Here's the drawing with two shaded views (mm, measured from the low corner). I have some questions. A direction names the side the tool comes from. Round coordinates to 2 decimals unless told otherwise and drop trailing zeros. Order: outer loops, then holes, each group sorted by start corner. A loop starts at its lowest first (then second) coordinate and runs counter-clockwise, first axis right, second up.
Q1. Will these pins go through, and if not, where does the flat tip stop? P1, Ø6.5, axis at x = 14.5, z = 74, coming from the +Y side; P2, Ø20.5, axis at y = 65.5, z = 60.5, coming from the +X side; P3, Ø11, axis at x = 93, y = 63.5, coming from the +Z side.
Q2. If we section it at A-A (z = 94): Please give me the cut outline in (x, y).
Q3. If we section it at D-D (x = 32.5): Please give me the cut outline in (y, z).
Q4. We'd pull the mould along X, two halves only. Please class the marked faces 1, 2 and 3: pulls with the +X half, pulls with the -X half, needs draft (parallel to the pull), parting line crosses it, or undercut.
Q5. For the marked faces 4 and 5, which set-ups out of +Z, -Z, +X, -X, +Y, -Y let a thin tool reach every point of the face, with its end or its side?
Q6. If we section it at C-C (x = 50.8): Please give me the cut outline in (y, z), plus the area to 3 significant figures.
Q7. If we section it at B-B (x = 89): Please give me the cut outline in (y, z).
Q8. If I drill on line 1 (X direction, y = 53, z = 64); line 2 (Y direction, x = 15, z = 39); line 3 (X direction, y = 70, z = 19.5), over which ranges is the centre line in solid material (lowest first)?
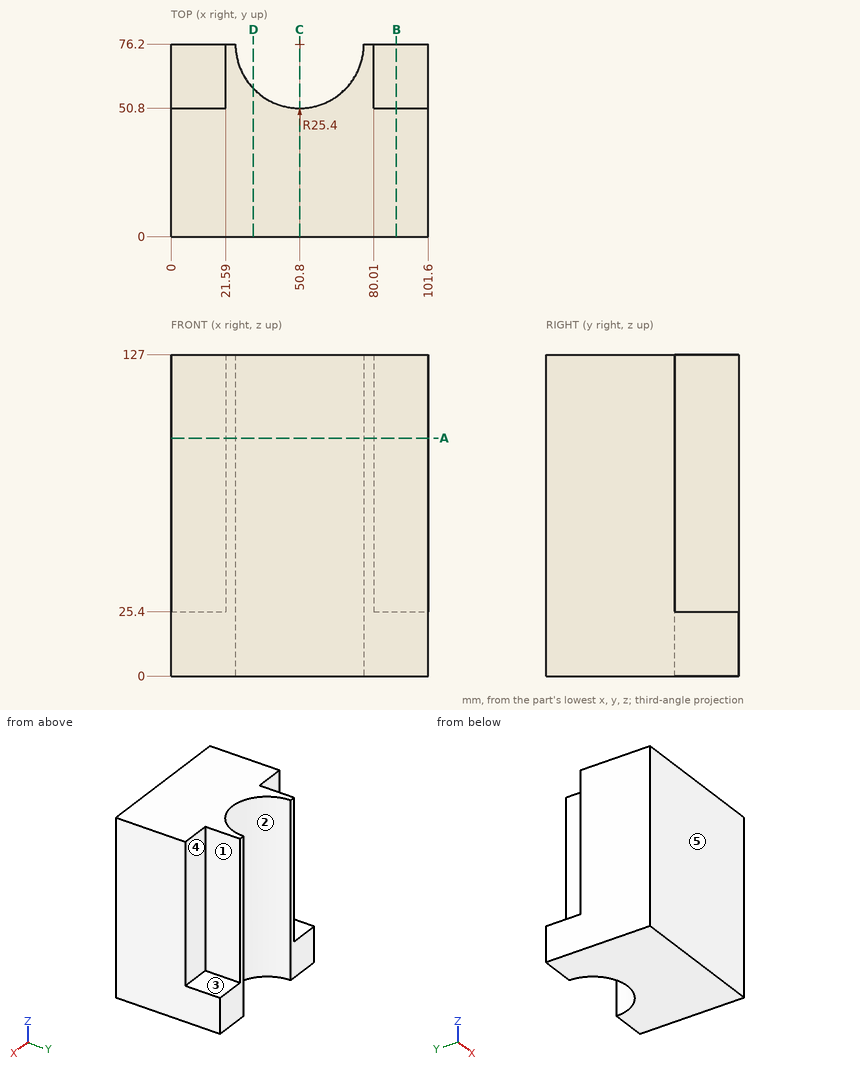
Solution:
1. P1: stops at y = 50.8
1. P2: stops at x = 80.01
1. P3: stops at z = 25.4
2. outline: (0, 0) - (101.6, 0) - (101.6, 50.8) - (80.01, 50.8) - (80.01, 76.2) - (76.2, 76.2) arc R25.4 cw to (25.4, 76.2) - (21.59, 76.2) - (21.59, 50.8) - (0, 50.8) - close
3. outline: (0, 0) - (58.59, 0) - (58.59, 127) - (0, 127) - close
4. face 1: pulls with the +X half
4. face 2: undercut
4. face 3: needs draft
5. face 4: +Z, +X, +Y
5. face 5: +Z, -Z, +X, -X, -Y
6. outline: (0, 0) - (50.8, 0) - (50.8, 127) - (0, 127) - close
6. area: 6,450 mm2
7. outline: (0, 0) - (76.2, 0) - (76.2, 25.4) - (50.8, 25.4) - (50.8, 127) - (0, 127) - close
8. line 1: x = 21.59 to 40.46, 61.14 to 80.01
8. line 2: y = 0 to 50.8
8. line 3: x = 0 to 26.17, 75.43 to 101.6
